Work out the finished part from the listing and answer in its coordinate system (mm). A direction names the side the tool comes from. Give positions to 0.01 mm unless a question says otherwise; leave off trailing zeros. Order: outer loops, then holes, each group sorted by start corner. A loop starts at its lowest first (then second) coordinate and runs counter-clockwise, first axis right, second up. Notation, with made-up numbers: (-40, -9) -> (6, -9) arc R6 cw to (6, -3) -> close; hole circle Ø1 at (34.5, 61.25). An arc over 180 degrees is marked (long way). Answer as CSV lines item,"result". Start each with the question number.
1. For faces 1 (the cylindrical face through (-39.916, 22.096, -0.249)), 2 (the flat face through (40.64, 11, 0)), 3 (the flat face through (21.129, 22, 10)), determine the directions among +Z, -Z, +X, -X, +Y, -Y from which every point of the face is accessible in a straight line to the end or side of a thin tool.
2. Find the intervals of material crossed by L1, parallel to Y at x = -17, z = 18; L2, parallel to X at y = 21.75, z = 12.5; L3, parallel to Y at x = -42, z = 5, in increasing order.
3. A cutting plane is placed at A-A (z = 14). Give the vertices of the cut face in (x, y).
4. For a pull along X with two mould halves and no side action, classify faces 4 (the flat face through (-1, 10, -20.32)), 5 (the cylindrical face through (51.812, 1.417, -16.331)), 6 (the flat face through (-25, 20.32, -4)) as released by +X, released by -X, zero draft, split by the parting line, or undercut.
5. Flat-ended cylindrical pins translate along their axes: pin 1 (3 mm diameter, centred on x = 14.5, z = 10, fed in from +Y); pin 2 (2 mm diameter, centred on y = 21.5, z = 9.5, fed in from -X); pin 3 (4 mm diameter, centred on x = -50, z = -2, fed in from +Y). Find the tip coordinate at first contact, or state that the pin passes through.
6. A cutting plane is placed at B-B (x = 18.5). Give the vertices of the cut face in (y, z), then the cut area to 3 significant figures.
7. A cutting plane is placed at C-C (y = 11.5). Give the vertices of the cut face in (x, z), then the cut area to 3 significant figures.
from build123d import *

# Parameters (mm, degrees)
SKETCH1_W            = 81.28
SKETCH1_H            = 40.64
BOSS_EXTRUDE1_DEPTH  = 22.86
FILLET1_R            = 2.54
SKETCH2_W            = 12.7
SKETCH2_H            = 35.56
BOSS_EXTRUDE2_DEPTH  = 2.794
FILLET2_R            = 5.08
SKETCH3_R            = 2.286
CUT_EXTRUDE1_DEPTH   = 61.503738364
FILLET2_OF_MIRROR1_R = 5.08
SKETCH4_W            = 7.230266788
SKETCH4_H            = 7.631948276
SKETCH4_W_2          = 9.652
SKETCH4_H_2          = 9.652
CUT_EXTRUDE2_DEPTH   = 2.54


with BuildPart() as part:
    # Sketch1 → Boss-Extrude1 (new body)
    with BuildSketch(Plane(origin=(0, 0, 0), x_dir=(1, 0, 0), z_dir=(0, 1, 0))):
        Rectangle(SKETCH1_W, SKETCH1_H)
    extrude(amount=BOSS_EXTRUDE1_DEPTH)

    # Fillet1
    fillet1_edges = [part.edges().sort_by_distance(p)[0] for p in [
        (-40.64, 22.86, 0),
        (0, 22.86, 20.32),
        (40.64, 22.86, 0),
        (0, 22.86, -20.32),
        (40.64, 11.43, 20.32),
        (-40.64, 11.43, 20.32),
        (-40.64, 11.43, -20.32),
        (40.64, 11.43, -20.32),
    ]]
    fillet(fillet1_edges, radius=FILLET1_R)

    # Sketch2 → Boss-Extrude2 (add)
    with BuildSketch(Plane.XZ):
        with Locations((46.99, 0)):
            Rectangle(SKETCH2_W, SKETCH2_H)
    boss_extrude2 = extrude(amount=-BOSS_EXTRUDE2_DEPTH)

    # Fillet2
    fillet2_edges = [part.edges().sort_by_distance(p)[0] for p in [
        (53.34, 1.397, 17.78),
        (53.34, 1.397, -17.78),
    ]]
    fillet(fillet2_edges, radius=FILLET2_R)

    # Sketch3 → Cut-Extrude1 (cut, through all)
    with BuildSketch(Plane(origin=(0, 2.794, 0), x_dir=(1, 0, 0), z_dir=(0, 1, 0))):
        with Locations(Location((48.514, 12.7, 0), (0, 0, 270))):
            Circle(SKETCH3_R)
        with Locations(Location((48.514, -12.7, 0), (0, 0, 270))):
            Circle(SKETCH3_R)
    cut_extrude1 = extrude(amount=-CUT_EXTRUDE1_DEPTH, mode=Mode.SUBTRACT)

    # Mirror1: Boss-Extrude2, Cut-Extrude1 across plane
    add(boss_extrude2.mirror(Plane(origin=(0, 0, 0), x_dir=(0, 0, 1), z_dir=(1, 0, 0))))
    add(cut_extrude1.mirror(Plane(origin=(0, 0, 0), x_dir=(0, 0, 1), z_dir=(1, 0, 0))), mode=Mode.SUBTRACT)

    # Fillet2 of Mirror1
    fillet2_of_mirror1_edges = [part.edges().sort_by_distance(p)[0] for p in [
        (-53.34, 1.397, 17.78),
        (-53.34, 1.397, -17.78),
    ]]
    fillet(fillet2_of_mirror1_edges, radius=FILLET2_OF_MIRROR1_R)

    # Sketch4 → Cut-Extrude2 (cut)
    with BuildSketch(Plane(origin=(0, 22.86, 0), x_dir=(1, 0, 0), z_dir=(0, 1, 0))):
        with Locations((-24.473297313, 3.624026455)):
            Rectangle(SKETCH4_W, SKETCH4_H)
        with Locations((16.303343502, -10.232970532)):
            Rectangle(SKETCH4_W_2, SKETCH4_H_2)
        with Locations((27.032885284, -10.232970532)):
            Rectangle(SKETCH4_W_2, SKETCH4_H_2)
    extrude(amount=-CUT_EXTRUDE2_DEPTH, mode=Mode.SUBTRACT)


solid = part.part
Answer sheet:
1,face 1,"+Z, -Z, -X, +Y"
1,face 2,"+Z, -Z, +X, +Y"
1,face 3,"+Y"
2,L1,"y = 0 to 22.85"
2,L2,"x = -40.2 to 11.48, 21.13 to 22.21, 31.86 to 40.2"
2,L3,"y = 0 to 2.79"
3,outline,"(-53.17, 0) -> (-50.39, 0) -> (-50.39, 2.79) -> (-53.17, 2.79) -> close; (-46.63, 0) -> (46.63, 0) -> (46.63, 2.79) -> (40.64, 2.79) -> (40.64, 20.32) arc R2.54 ccw to (38.1, 22.86) -> (31.86, 22.86) -> (31.86, 20.32) -> (22.21, 20.32) -> (22.21, 22.86) -> (21.13, 22.86) -> (21.13, 20.32) -> (11.48, 20.32) -> (11.48, 22.86) -> (-38.1, 22.86) arc R2.54 ccw to (-40.64, 20.32) -> (-40.64, 2.79) -> (-46.63, 2.79) -> close; (50.39, 0) -> (53.17, 0) -> (53.17, 2.79) -> (50.39, 2.79) -> close"
4,face 4,"zero draft"
4,face 5,"released by +X"
4,face 6,"undercut"
5,pin 1,"stops at y = 20.32"
5,pin 2,"stops at x = -40.63"
5,pin 3,"stops at y = 2.79"
6,outline,"(0, -20.32) -> (20.32, -20.32) arc R2.54 ccw to (22.86, -17.78) -> (22.86, 5.41) -> (20.32, 5.41) -> (20.32, 15.06) -> (22.86, 15.06) -> (22.86, 17.78) arc R2.54 ccw to (20.32, 20.32) -> (0, 20.32) -> close"
6,area,"902 mm^2"
7,outline,"(-40.64, -17.78) arc R2.54 ccw to (-38.1, -20.32) -> (38.1, -20.32) arc R2.54 ccw to (40.64, -17.78) -> (40.64, 17.78) arc R2.54 ccw to (38.1, 20.32) -> (-38.1, 20.32) arc R2.54 ccw to (-40.64, 17.78) -> close"
7,area,"3,300 mm^2"
